Model file for the job. Use its own axes, mm. Round coordinates to 2 decimals unless told otherwise and drop trailing zeros. Loops run counter-clockwise (first coordinate to the right, second up) from the corner with the lowest first, then second, coordinate; pieces in that order, holes last. Notation, with made-up numbers: M 21,45 L 30,45 A20 ccw 30,65 Z; hole C 21.5,26.5 d4. An arc over 180 degrees is marked long. Use a Markdown table: item, result. Add a question column.
Item 1: Saw through at C-C on y = 0.85. Write the cut outline in (x, z), then the cut area to 3 significant figures.
Item 2: Saw through at B-B on x = 0. Write the cut outline in (y, z), then the cut area to 3 significant figures.
Item 3: Saw through at D-D on z = 25. Write the cut outline in (x, y).
Item 4: Saw through at A-A on z = 0. Write the cut outline in (x, y), then the cut area to 3 significant figures.
Item 5: Wall check: L1, parallel to X at y = 0.75, z = 0; L2, parallel to X at y = 0.7, z = 1. Give the ranges that are in metal, low to high. Write a range as from..to.
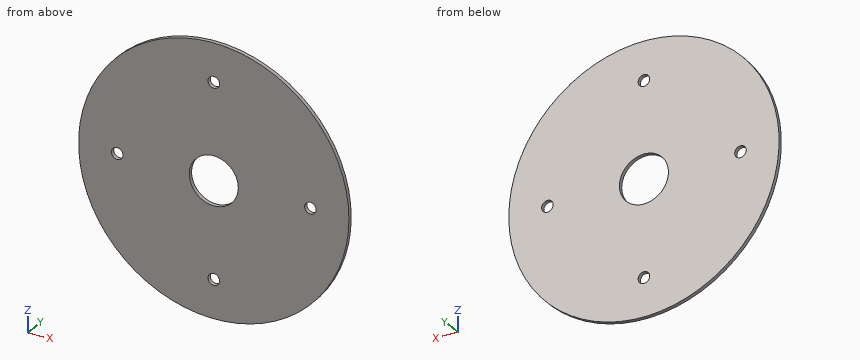
```python
from build123d import *

# Parameters (mm, degrees)
SKETCH1_R           = 35
BOSS_EXTRUDE1_DEPTH = 1
SKETCH2_R           = 6.35
CUT_EXTRUDE1_DEPTH  = 1
SKETCH3_R           = 1.5
CUT_EXTRUDE4_DEPTH  = 1
CIRPATTERN1_COUNT   = 4


with BuildPart() as part:
    # Sketch1 → Boss-Extrude1 (new body)
    with BuildSketch(Plane(origin=(0, 0, 0), x_dir=(1, 0, 0), z_dir=(0, 1, 0))):
        Circle(SKETCH1_R)
    extrude(amount=BOSS_EXTRUDE1_DEPTH)

    # Sketch2 → Cut-Extrude1 (cut)
    with BuildSketch(Plane(origin=(0, 1, 0), x_dir=(1, 0, 0), z_dir=(0, 1, 0))):
        Circle(SKETCH2_R)
    extrude(amount=-CUT_EXTRUDE1_DEPTH, mode=Mode.SUBTRACT)

    # Sketch3 → Cut-Extrude4 (cut)
    with BuildSketch(Plane(origin=(0, 1, 0), x_dir=(1, 0, 0), z_dir=(0, 1, 0))):
        with Locations((0, 25)):
            Circle(SKETCH3_R)
    cut_extrude4 = extrude(amount=-CUT_EXTRUDE4_DEPTH, mode=Mode.SUBTRACT)

    # CirPattern1: Cut-Extrude4 ×4 about axis
    cirpattern1_axis = Axis((0, 0, 0), (0, 1, 0))
    for i in range(1, CIRPATTERN1_COUNT):
        add(cut_extrude4.rotate(cirpattern1_axis, i * 360 / CIRPATTERN1_COUNT), mode=Mode.SUBTRACT)


solid = part.part
```
Entries:
| question | item | result |
|---|---|---|
| 1 | outline | C 0,0 d70; hole C -25,0 d3; hole C 0,0 d12.7; hole C 0,-25 d3; hole C 0,25 d3; hole C 25,0 d3 |
| 1 | area | 3,690 mm2 |
| 2 | outline | M 0,-35 L 1,-35 L 1,-26.5 L 0,-26.5 Z; M 0,-23.5 L 1,-23.5 L 1,-6.35 L 0,-6.35 Z; M 0,6.35 L 1,6.35 L 1,23.5 L 0,23.5 Z; M 0,26.5 L 1,26.5 L 1,35 L 0,35 Z |
| 2 | area | 51.3 mm2 |
| 3 | outline | M -24.49,0 L -1.5,0 L -1.5,1 L -24.49,1 Z; M 1.5,0 L 24.49,0 L 24.49,1 L 1.5,1 Z |
| 4 | outline | M -35,0 L -26.5,0 L -26.5,1 L -35,1 Z; M -23.5,0 L -6.35,0 L -6.35,1 L -23.5,1 Z; M 6.35,0 L 23.5,0 L 23.5,1 L 6.35,1 Z; M 26.5,0 L 35,0 L 35,1 L 26.5,1 Z |
| 4 | area | 51.3 mm2 |
| 5 | L1 | -35..-26.5, -23.5..-6.35, 6.35..23.5, 26.5..35 |
| 5 | L2 | -34.99..-26.12, -23.88..-6.27, 6.27..23.88, 26.12..34.99 |
